Build history of the part. All positions in model axes, mm. A direction names the side the tool comes from. Give positions to 0.01 mm unless a question says otherwise; leave off trailing zeros. Order: outer loops, then holes, each group sorted by start corner. A loop starts at its lowest first (then second) coordinate and runs counter-clockwise, first axis right, second up. Notation, with made-up numbers: (9, 77.25) - (41, 77.25) arc R22 ccw to (41, 104.25) - close; hole circle Ø10 at (-26.5, 72.25). An arc over 180 degrees is marked (long way). Answer in a Markdown table with one row per item.
```python
from build123d import *

# Parameters (mm, degrees)
SKETCH1_R           = 1.015999988
SKETCH1_R_2         = 1.5
BOSS_EXTRUDE1_DEPTH = 1.397


with BuildPart() as part:
    # Sketch1 → Boss-Extrude1 (new body)
    with BuildSketch(Plane(origin=(0, 0, 0), x_dir=(1, 0, 0), z_dir=(0, 1, 0))):
        with BuildLine():
            Line((-44.657487237, -41.209177315), (-46.396043568, -42.947733628))
            ThreePointArc((-46.396043568, -42.947733628), (-46.470434263, -43.125880965), (-46.398093324, -43.304870455))
            Line((-46.398093324, -43.304870455), (-43.050556795, -46.730153534))
            ThreePointArc((-43.050556795, -46.730153534), (-42.865374809, -46.831022569), (-42.667823867, -46.757262447))
            Line((-42.667823867, -46.757262447), (-40.871772634, -44.961211232))
            ThreePointArc((-40.871772634, -44.961211232), (-38.831009245, -46.687575098), (-36.702263685, -48.30420423))
            ThreePointArc((-36.702263685, -48.30420423), (-33.138347002, -49.294565873), (-29.78114627, -47.741658512))
            ThreePointArc((-29.78114627, -47.741658512), (0, -32.054645119), (29.78114627, -47.741658512))
            ThreePointArc((29.78114627, -47.741658512), (33.138347002, -49.294565873), (36.702263685, -48.30420423))
            ThreePointArc((36.702263685, -48.30420423), (38.831009245, -46.687575098), (40.871772634, -44.961211232))
            Line((40.871772634, -44.961211232), (42.667823867, -46.757262447))
            ThreePointArc((42.667823867, -46.757262447), (42.865374809, -46.831022569), (43.050556795, -46.730153534))
            Line((43.050556795, -46.730153534), (46.398093324, -43.304870455))
            ThreePointArc((46.398093324, -43.304870455), (46.470434263, -43.125880965), (46.396043568, -42.947733628))
            Line((46.396043568, -42.947733628), (44.657487237, -41.209177315))
            ThreePointArc((44.657487237, -41.209177315), (46.545191357, -39.007785017), (48.30420423, -36.702263685))
            ThreePointArc((48.30420423, -36.702263685), (49.294565905, -33.13834702), (47.741658512, -29.78114627))
            ThreePointArc((47.741658512, -29.78114627), (41.575395348, 0), (47.741658512, 29.78114627))
            ThreePointArc((47.741658512, 29.78114627), (49.294565905, 33.13834702), (48.30420423, 36.702263685))
            ThreePointArc((48.30420423, 36.702263685), (46.545191357, 39.007785017), (44.657487237, 41.209177315))
            Line((44.657487237, 41.209177315), (46.396043568, 42.947733628))
            ThreePointArc((46.396043568, 42.947733628), (46.470434263, 43.125880965), (46.398093324, 43.304870455))
            Line((46.398093324, 43.304870455), (43.050556795, 46.730153534))
            ThreePointArc((43.050556795, 46.730153534), (42.865374809, 46.831022569), (42.667823867, 46.757262447))
            Line((42.667823867, 46.757262447), (40.871772634, 44.961211232))
            ThreePointArc((40.871772634, 44.961211232), (38.831009245, 46.687575098), (36.702263685, 48.30420423))
            ThreePointArc((36.702263685, 48.30420423), (33.138347002, 49.294565873), (29.78114627, 47.741658512))
            ThreePointArc((29.78114627, 47.741658512), (0, 32.054645119), (-29.78114627, 47.741658512))
            ThreePointArc((-29.78114627, 47.741658512), (-33.138347002, 49.294565873), (-36.702263685, 48.30420423))
            ThreePointArc((-36.702263685, 48.30420423), (-38.831009245, 46.687575098), (-40.871772634, 44.961211232))
            Line((-40.871772634, 44.961211232), (-42.667823867, 46.757262447))
            ThreePointArc((-42.667823867, 46.757262447), (-42.865374809, 46.831022569), (-43.050556795, 46.730153534))
            Line((-43.050556795, 46.730153534), (-46.398093324, 43.304870455))
            ThreePointArc((-46.398093324, 43.304870455), (-46.470434263, 43.125880965), (-46.396043568, 42.947733628))
            Line((-46.396043568, 42.947733628), (-44.657487237, 41.209177315))
            ThreePointArc((-44.657487237, 41.209177315), (-46.545191357, 39.007785017), (-48.30420423, 36.702263685))
            ThreePointArc((-48.30420423, 36.702263685), (-49.294565905, 33.13834702), (-47.741658512, 29.78114627))
            ThreePointArc((-47.741658512, 29.78114627), (-41.575395348, 0), (-47.741658512, -29.78114627))
            ThreePointArc((-47.741658512, -29.78114627), (-49.294565905, -33.13834702), (-48.30420423, -36.702263685))
            ThreePointArc((-48.30420423, -36.702263685), (-46.545191357, -39.007785017), (-44.657487237, -41.209177315))
        make_face()
        with Locations(Location((-35.273880272, -43.89492624, 0), (0, 0, 90))):
            Circle(SKETCH1_R, mode=Mode.SUBTRACT)
        with Locations(Location((-43.894926149, -35.273880364, 0), (0, 0, 270))):
            Circle(SKETCH1_R, mode=Mode.SUBTRACT)
        with Locations(Location((-31.299173944, -31.299174035, 0), (0, 0, 270))):
            Circle(SKETCH1_R, mode=Mode.SUBTRACT)
        with Locations(Location((43.894926149, -35.273880364, 0), (0, 0, 90))):
            Circle(SKETCH1_R, mode=Mode.SUBTRACT)
        with Locations(Location((35.273880272, -43.89492624, 0), (0, 0, 270))):
            Circle(SKETCH1_R, mode=Mode.SUBTRACT)
        with Locations(Location((31.299173944, -31.299174035, 0), (0, 0, 90))):
            Circle(SKETCH1_R, mode=Mode.SUBTRACT)
        with Locations(Location((-35.273880272, 43.89492624, 0), (0, 0, 270))):
            Circle(SKETCH1_R, mode=Mode.SUBTRACT)
        with Locations(Location((-31.299173944, 31.299174035, 0), (0, 0, 90))):
            Circle(SKETCH1_R, mode=Mode.SUBTRACT)
        with Locations(Location((-43.894926149, 35.273880364, 0), (0, 0, 90))):
            Circle(SKETCH1_R, mode=Mode.SUBTRACT)
        with Locations(Location((43.894926149, 35.273880364, 0), (0, 0, 270))):
            Circle(SKETCH1_R, mode=Mode.SUBTRACT)
        with Locations(Location((35.273880272, 43.89492624, 0), (0, 0, 90))):
            Circle(SKETCH1_R, mode=Mode.SUBTRACT)
        with Locations(Location((31.299173944, 31.299174035, 0), (0, 0, 270))):
            Circle(SKETCH1_R, mode=Mode.SUBTRACT)
        with Locations(Location((-39, 24.5, 0), (0, 0, 270))):
            Circle(SKETCH1_R_2, mode=Mode.SUBTRACT)
        with Locations(Location((19, 24.5, 0), (0, 0, 270))):
            Circle(SKETCH1_R_2, mode=Mode.SUBTRACT)
        with Locations(Location((19.002972949, -24.499403884, 0), (0, 0, 270))):
            Circle(SKETCH1_R_2, mode=Mode.SUBTRACT)
        with Locations(Location((-39, -24.5, 0), (0, 0, 270))):
            Circle(SKETCH1_R_2, mode=Mode.SUBTRACT)
    extrude(amount=BOSS_EXTRUDE1_DEPTH)


solid = part.part
```
1. Cut at C-C on x = -17.5. Write the cut outline in (y, z), and give its area (3 significant figures).
Check result:
| item | result |
|---|---|
| outline | (0, -36.58) - (1.4, -36.58) - (1.4, 36.58) - (0, 36.58) - close |
| area | 102 mm² |
2. Cut at B-B on z = -24.5. Write the cut outline in (x, y), and give its area (3 significant figures).
Check result:
| item | result |
|---|---|
| outline | (-45.69, 0) - (-40.5, 0) - (-40.5, 1.4) - (-45.69, 1.4) - close; (-37.5, 0) - (17.5, 0) - (17.5, 1.4) - (-37.5, 1.4) - close; (20.5, 0) - (45.69, 0) - (45.69, 1.4) - (20.5, 1.4) - close |
| area | 119 mm² |
3. Two-plate mould, pull along Z, no slides. Class faces 5 (the face through (-41.577, 0.689, -0.429)), 6 (the face through (-1, 1.397, -1)), 7 (the face through (46.52, 0.69, 39.04)), 8 (the face through (44.7, 0.69, 45.04)): +Z half, -Z half, draft (parallel to the pull), parting line (faces both ways), or undercut.
Check result:
| item | result |
|---|---|
| face 5 | undercut |
| face 6 | draft |
| face 7 | undercut |
| face 8 | +Z half |
4. Probe line 1 (Z direction, x = -34.5, y = 0.25); line 2 (X direction, y = 1.25, z = 43.5); line 3 (X direction, y = 0.9, z = 39). List the from-to ranges inside material, lowest first.
Check result:
| item | result |
|---|---|
| line 1 | z = -49.23 to -44.55, -43.24 to 43.24, 44.55 to 49.23 |
| line 2 | x = -46.21 to -36.21, -34.34 to -26.38, 26.38 to 34.34, 36.21 to 46.21 |
| line 3 | x = -46.55 to -21.29, 21.29 to 46.55 |
5. Cut at D-D on y = 0.4. Count the separate pieces of the cut face and the enclosed holes in it, and give its area (3 significant figures).
Check result:
| item | result |
|---|---|
| separate pieces | 1 |
| enclosed holes | 16 |
| area | 7,180 mm² |
6. Which spindle directions (+Z, -Z, +X, -X, +Y, -Y) get a long thin tool onto all of the face, cutting with end or side? Do faces 1 (the face through (46.57, 0.69, -38.98)), 2 (the face through (38.8, 0.69, 46.71)), 3 (the face through (-46.52, 0.69, -39.04)), 4 (the face through (-38.8, 0.69, -46.71)). Say none if no direction does.
Check result:
| item | result |
|---|---|
| face 1 | +X, +Y, -Y |
| face 2 | +Z, +Y, -Y |
| face 3 | -X, +Y, -Y |
| face 4 | -Z, +Y, -Y |
7. Cut at A-A on x = -39. Write the cut outline in (y, z).
Check result:
| item | result |
|---|---|
| outline | (0, -46.55) - (1.4, -46.55) - (1.4, -26) - (0, -26) - close; (0, -23) - (1.4, -23) - (1.4, 23) - (0, 23) - close; (0, 26) - (1.4, 26) - (1.4, 46.55) - (0, 46.55) - close |
